```python
from build123d import *

# Parameters (mm, degrees)
SKETCH1_W               = 31.2625
SKETCH1_H               = 55
BOSS_EXTRUDE1_DEPTH     = 3.175
SKETCH2_R               = 1.5
CUT_EXTRUDE1_DEPTH      = 10
LPATTERN1_COUNT         = 3
LPATTERN1_PITCH         = 10
LPATTERN1_COL_COUNT     = 3
LPATTERN1_COL_PITCH     = 10
SKETCH3_W               = 6.35
SKETCH3_H               = 3.175
CUT_EXTRUDE2_DEPTH      = 10
LPATTERN2_COUNT         = 5
LPATTERN2_PITCH         = 6.35
LPATTERN2_COL_COUNT     = 5
LPATTERN2_COL_PITCH     = 6.35
SKETCH4_W               = 3.175
SKETCH4_H               = 3.6875
SKETCH4_H_2             = 3.175
CUT_EXTRUDE3_DEPTH      = 10
SKETCH5_W               = 6.35
SKETCH5_H               = 55
CUT_EXTRUDE4_DEPTH      = 10
SKETCH6_W               = 3.175
SKETCH6_H               = 3.175
CUT_EXTRUDE5_DEPTH      = 10
LPATTERN3_COUNT         = 2
LPATTERN3_PITCH         = 6.35
LPATTERN3_COUNT_DIR2    = 2
LPATTERN3_PITCH_DIR2    = 6.35
SKETCH7_W               = 5.8625
SKETCH7_H               = 3.175
CUT_EXTRUDE6_DEPTH      = 10
MIRROR1_COPY_1_SKETCH_W = 3.175
MIRROR1_COPY_1_SKETCH_H = 3.175
MIRROR1_COPY_1_DEPTH    = 10
MIRROR1_COPY_2_SKETCH_W = 3.175
MIRROR1_COPY_2_SKETCH_H = 3.175
MIRROR1_COPY_2_DEPTH    = 10
MIRROR1_COPY_3_SKETCH_W = 3.175
MIRROR1_COPY_3_SKETCH_H = 3.175
MIRROR1_COPY_3_DEPTH    = 10


with BuildPart() as part:
    # Sketch1 → Boss-Extrude1 (new body)
    with BuildSketch(Plane.XY):
        Rectangle(SKETCH1_W, SKETCH1_H)
    extrude(amount=BOSS_EXTRUDE1_DEPTH)

    # Sketch2 → Cut-Extrude1 (cut)
    with BuildSketch(Plane.XY.offset(3.175)):
        Circle(SKETCH2_R)
    cut_extrude1 = extrude(amount=-CUT_EXTRUDE1_DEPTH, mode=Mode.SUBTRACT)

    # LPattern1: Cut-Extrude1 ×3
    with Locations(*[(0, i * LPATTERN1_PITCH, 0) for i in range(1, LPATTERN1_COUNT)]):
        add(cut_extrude1, mode=Mode.SUBTRACT)

    # LPattern1 col: Cut-Extrude1 ×3
    with Locations(*[(0, -i * LPATTERN1_COL_PITCH, 0) for i in range(1, LPATTERN1_COL_COUNT)]):
        add(cut_extrude1, mode=Mode.SUBTRACT)

    # Sketch3 → Cut-Extrude2 (cut)
    with BuildSketch(Plane.XY.offset(3.175)):
        with Locations((15.63125, -3.175)):
            Rectangle(SKETCH3_W, SKETCH3_H)
    cut_extrude2 = extrude(amount=-CUT_EXTRUDE2_DEPTH, mode=Mode.SUBTRACT)

    # LPattern2: Cut-Extrude2 ×5
    with Locations(*[(0, i * LPATTERN2_PITCH, 0) for i in range(1, LPATTERN2_COUNT)]):
        add(cut_extrude2, mode=Mode.SUBTRACT)

    # LPattern2 col: Cut-Extrude2 ×5
    with Locations(*[(0, -i * LPATTERN2_COL_PITCH, 0) for i in range(1, LPATTERN2_COL_COUNT)]):
        add(cut_extrude2, mode=Mode.SUBTRACT)

    # Sketch4 → Cut-Extrude3 (cut)
    with BuildSketch(Plane.XY.offset(3.175)):
        with Locations((14.04375, 25.65625)):
            Rectangle(SKETCH4_W, SKETCH4_H)
        with Locations((14.04375, -25.4)):
            Rectangle(SKETCH4_W, SKETCH4_H_2)
    extrude(amount=-CUT_EXTRUDE3_DEPTH, mode=Mode.SUBTRACT)

    # Sketch5 → Cut-Extrude4 (cut)
    with BuildSketch(Plane.XY.offset(3.175)):
        with Locations((-12.45625, 0)):
            Rectangle(SKETCH5_W, SKETCH5_H)
    extrude(amount=-CUT_EXTRUDE4_DEPTH, mode=Mode.SUBTRACT)

    # Sketch6 → Cut-Extrude5 (cut)
    with BuildSketch(Plane.XY.offset(3.175)):
        with Locations((-4.51875, 25.9125)):
            Rectangle(SKETCH6_W, SKETCH6_H)
    cut_extrude5 = extrude(amount=-CUT_EXTRUDE5_DEPTH, mode=Mode.SUBTRACT)

    # LPattern3: Cut-Extrude5 2 × 2
    with Locations(*[(i * LPATTERN3_PITCH, j * LPATTERN3_PITCH_DIR2, 0) for i in range(LPATTERN3_COUNT) for j in range(LPATTERN3_COUNT_DIR2) if (i, j) != (0, 0)]):
        add(cut_extrude5, mode=Mode.SUBTRACT)

    # Sketch7 → Cut-Extrude6 (cut)
    with BuildSketch(Plane.XY.offset(3.175)):
        with Locations((9.525, 25.9125)):
            Rectangle(SKETCH7_W, SKETCH7_H)
    cut_extrude6 = extrude(amount=-CUT_EXTRUDE6_DEPTH, mode=Mode.SUBTRACT)

    # Mirror1: Cut-Extrude5, Cut-Extrude6 across plane
    add(cut_extrude5.mirror(Plane.ZX), mode=Mode.SUBTRACT)
    add(cut_extrude6.mirror(Plane.ZX), mode=Mode.SUBTRACT)

    # Mirror1 copy 1 sketch → Mirror1 copy 1 (cut)
    with BuildSketch(Plane(origin=(0, -6.35, 3.175), x_dir=(1, 0, 0), z_dir=(0, 0, 1))):
        with Locations((-4.51875, -25.9125)):
            Rectangle(MIRROR1_COPY_1_SKETCH_W, MIRROR1_COPY_1_SKETCH_H)
    extrude(amount=-MIRROR1_COPY_1_DEPTH, mode=Mode.SUBTRACT)

    # Mirror1 copy 2 sketch → Mirror1 copy 2 (cut)
    with BuildSketch(Plane(origin=(6.35, 0, 3.175), x_dir=(1, 0, 0), z_dir=(0, 0, 1))):
        with Locations((-4.51875, -25.9125)):
            Rectangle(MIRROR1_COPY_2_SKETCH_W, MIRROR1_COPY_2_SKETCH_H)
    extrude(amount=-MIRROR1_COPY_2_DEPTH, mode=Mode.SUBTRACT)

    # Mirror1 copy 3 sketch → Mirror1 copy 3 (cut)
    with BuildSketch(Plane(origin=(6.35, -6.35, 3.175), x_dir=(1, 0, 0), z_dir=(0, 0, 1))):
        with Locations((-4.51875, -25.9125)):
            Rectangle(MIRROR1_COPY_3_SKETCH_W, MIRROR1_COPY_3_SKETCH_H)
    extrude(amount=-MIRROR1_COPY_3_DEPTH, mode=Mode.SUBTRACT)


solid = part.part
```
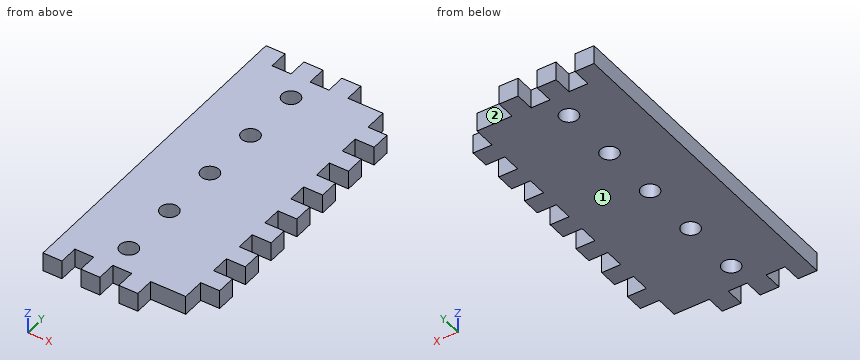
Check sheet for the modelled part. Datum: model origin and axes. Units: mm. Face numbers are marked on the shaded views. A direction names the side the tool comes from. Give positions to 0.01 mm unless a question says otherwise; leave off trailing zeros. Write each loop counter-clockwise with the first axis right and the second up, starting at its lowest first coordinate (ties: lowest second). Pieces come first, ordered by that corner, then holes.
Item 1: Gauge pin test, flat ends, axial feed: pin 1 (1.6 mm diameter, centred on x = 14, z = 2, fed in from -Y); pin 2 (1 mm diameter, centred on x = 1, z = 1, fed in from -Y) (3 decimals); pin 3 (1 mm diameter, centred on y = -25, z = 2.5, fed in from +X); pin 4 (2.5 mm diameter, centred on x = 0, y = -10, fed in from +Z). Record the tip position at first contact, or that the pin passes through.
Item 2: Cross-section at A-A (y = 10). Enter the section's corners in (x, z) (3 decimals).
Item 3: Scan lines: L1, parallel to Y at x = 0, z = 1.45; L2, parallel to Y at x = 8, z = 0.7 (3 decimals); L3, parallel to X at y = -4, z = 0.8. Record each from-to range of solid material in increasing order.
Item 4: Cross-section at D-D (x = 10.75). Enter the section's corners in (y, z) (3 decimals).
Item 5: Cross-section at C-C (z = 1.15). Count the separate pieces of the cut face and the enclosed holes in it, and give its area (3 significant figures).
Item 6: Access from +Z, -Z, +X, -X, +Y, -Y to the whole of each face (thin tool, end or side, straight path). Record for the marked faces 1 and 2.
Item 7: Cross-section at B-B (y = 20). Enter the section's corners in (x, z) (3 decimals), and give its area (3 significant figures).
Report:
1. pin 1: stops at y = -20.64
1. pin 2: stops at y = -24.325
1. pin 3: stops at x = 6.59
1. pin 4: passes through
2. outline: (-9.281, 0) - (-1.5, 0) - (-1.5, 3.175) - (-9.281, 3.175) - close; (1.5, 0) - (12.456, 0) - (12.456, 3.175) - (1.5, 3.175) - close
3. L1: y = -27.5 to -21.5, -18.5 to -11.5, -8.5 to -1.5, 1.5 to 8.5, 11.5 to 18.5, 21.5 to 27.5
3. L2: y = -24.325 to 24.325
3. L3: x = -9.28 to 12.46
4. outline: (-24.325, 0) - (24.325, 0) - (24.325, 3.175) - (-24.325, 3.175) - close
5. separate pieces: 1
5. enclosed holes: 5
5. area: 1,150 mm2
6. face 1: -Z, +X, -X, +Y, -Y
6. face 2: +Z, -Z, +X, +Y
7. outline: (-9.281, 0) - (-1.5, 0) - (-1.5, 3.175) - (-9.281, 3.175) - close; (1.5, 0) - (15.631, 0) - (15.631, 3.175) - (1.5, 3.175) - close
7. area: 69.6 mm2
